```python
from build123d import *

# Parameters (mm, degrees)
F0_W     = 1066.8
F0_H     = 2057.4
F0_W_2   = 1016
F0_H_2   = 2006.6
F1_DEPTH = 25.4
F2_W     = 304.8
F2_H     = 25.4
F3_DEPTH = 25.4
F4_W     = 25.4
F4_H     = 25.4
F5_DEPTH = 1778


with BuildPart() as f1:
    # F0 (on Front) → F1 (new body)
    with BuildSketch(Plane.XZ):
        Rectangle(F0_W, F0_H)
        Rectangle(F0_W_2, F0_H_2, mode=Mode.SUBTRACT)
    extrude(amount=F1_DEPTH)

    # F2 (on face) → F3 (join)
    with BuildSketch(Plane.YZ.offset(533.4)):
        with Locations((152.4, -101.6)):
            Rectangle(F2_W, F2_H)
    extrude(amount=-F3_DEPTH)

    # F4 (on face) → F5 (join)
    with BuildSketch(Plane(origin=(0, 0, 0), x_dir=(-1, 0, 0), z_dir=(0, 1, 0))):
        with Locations((-520.7, -1016)):
            Rectangle(F4_W, F4_H)
    extrude(amount=F5_DEPTH)


solid = f1.part
```
Read the model definition and answer for the solid it produces. Units are mm, in the model's axes. Round coordinates to 2 decimals unless told otherwise and drop trailing zeros. Write each loop counter-clockwise with the first axis right and the second up, starting at its lowest first coordinate (ties: lowest second). Pieces come first, ordered by that corner, then holes. Notation, with made-up numbers: (-19.5, -1) -> (3.5, -1) arc R16 cw to (3.5, 30) -> close; hole circle Ø7 at (14.25, 49). An arc over 180 degrees is marked (long way). Answer in a Markdown table with one row per item. Add a question column.
1) Find section C-C, the plane y = 504.5. Determine the outline of the cut face in (x, z).
2) Find section B-B, the plane x = 204.5. Determine the outline of the cut face in (y, z).
3) Find section A-A, the plane z = 337.5. Determine the outline of the cut face in (x, y), and give its area (3 significant figures).
4) Given P1, Ø12.5, axis at x = 524.5, z = -96, coming from the +Y side; P2, Ø12.5, axis at x = 524, y = 169, coming from the +Z side; P3, Ø20.5, axis at x = 515.5, z = -340.5, coming from the +Y side, each flat-ended and moving along its own axis, determine where each tip first touches the part or whether it passes through.
5) Determine the mould class of faces 1 (the face through (516, 872, -1028.7)), 2 (the face through (508, -19, -5)) for opening direction X: pulls with the +X half, pulls with the -X half, needs draft (parallel to the pull), parting line crosses it, or undercut.
Findings below:
| question | item | result |
|---|---|---|
| 1 | outline | (508, -1028.7) -> (533.4, -1028.7) -> (533.4, -1003.3) -> (508, -1003.3) -> close |
| 2 | outline | (-25.4, -1028.7) -> (0, -1028.7) -> (0, -1003.3) -> (-25.4, -1003.3) -> close; (-25.4, 1003.3) -> (0, 1003.3) -> (0, 1028.7) -> (-25.4, 1028.7) -> close |
| 3 | outline | (-533.4, -25.4) -> (-508, -25.4) -> (-508, 0) -> (-533.4, 0) -> close; (508, -25.4) -> (533.4, -25.4) -> (533.4, 0) -> (508, 0) -> close |
| 3 | area | 1,290 mm² |
| 4 | P1 | y = 304.8 |
| 4 | P2 | z = -88.9 |
| 4 | P3 | y = 0 |
| 5 | face 1 | needs draft |
| 5 | face 2 | undercut |
